Model file for the job. Use its own axes, mm. Round coordinates to 2 decimals unless told otherwise and drop trailing zeros. Loops run counter-clockwise (first coordinate to the right, second up) from the corner with the lowest first, then second, coordinate; pieces in that order, holes last. Notation, with made-up numbers: M 79.5,17 L 115.5,17 A19 cw 115.5,47 Z; hole C -10.5,-22 d2. An arc over 180 degrees is marked long. Use a Markdown table: item, result. Add a question column.
Item 1: Saw through at A-A on z = 2.5. Write the cut outline in (x, y), then the cut area to 3 significant figures.
Item 2: Pin check, flat tips, straight feed: P1, Ø1.2, axis at x = -10, y = 10.5, coming from the +Z side; P2, Ø1.5, axis at x = -10.86, y = 11.26, coming from the +Z side; P3, Ø4, axis at y = 7.5, z = 2, coming from the +X side; P4, Ø1.5, axis at x = 12, z = 6.5, coming from the -Y side. Stop position of each tip, or through.
Item 3: Saw through at B-B on x = -10.5. Write the cut outline in (y, z).
Item 4: Saw through at D-D on y = 5.5. Write the cut outline in (x, z).
Item 5: Saw through at C-C on z = 7.5. Write the cut outline in (x, y).
Item 6: Wall check: L1, parallel to X at y = 12.5, z = 7.75; L2, parallel to X at y = 11, z = 1.75; L3, parallel to Y at x = 20, z = 5.75. Give the ranges that are in metal, low to high. Write a range as from..to.
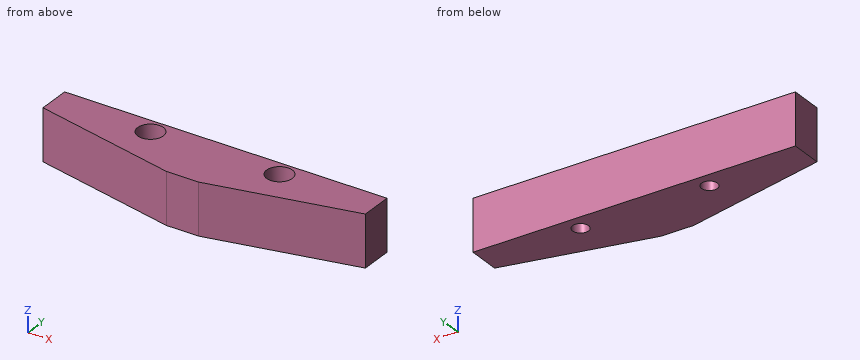
```python
from build123d import *

# Parameters (mm, degrees)
EXTRUDE_1_DEPTH     = 8
SKETCH_2_R          = 1.25
CUT_EXTRUDE_1_DEPTH = 8
SKETCH_3_R          = 2
CUT_EXTRUDE_2_DEPTH = 4


with BuildPart() as part:
    # Эскиз1 → Бобышка-Вытянуть1 (new body)
    with BuildSketch(Plane.XY):
        Polygon((-25.856072272, 13.757630696), (24.143927728, 13.757630696), (24.143927728, 8.757630696), (1.643927728, 3.757630696), (-3.356072272, 3.757630696), (-25.856072272, 8.757630696), align=None)
    extrude(amount=EXTRUDE_1_DEPTH)

    # Эскиз2 → Вырез-Вытянуть1 (cut)
    with BuildSketch(Plane.XY.offset(8)):
        with Locations((-10.856072272, 11.257630696)):
            Circle(SKETCH_2_R)
        with Locations((9.143927728, 11.257630696)):
            Circle(SKETCH_2_R)
    extrude(amount=-CUT_EXTRUDE_1_DEPTH, mode=Mode.SUBTRACT)

    # Эскиз3 → Вырез-Вытянуть2 (cut)
    with BuildSketch(Plane.XY.offset(8)):
        with Locations((-10.856072272, 11.257630696)):
            Circle(SKETCH_3_R)
        with Locations((9.143927728, 11.257630696)):
            Circle(SKETCH_3_R)
    extrude(amount=-CUT_EXTRUDE_2_DEPTH, mode=Mode.SUBTRACT)


solid = part.part
```
Entries:
| question | item | result |
|---|---|---|
| 1 | outline | M -25.86,8.76 L -3.36,3.76 L 1.64,3.76 L 24.14,8.76 L 24.14,13.76 L -25.86,13.76 Z; hole C -10.86,11.26 d2.5; hole C 9.14,11.26 d2.5 |
| 1 | area | 378 mm2 |
| 2 | P1 | z = 4 |
| 2 | P2 | through |
| 2 | P3 | x = 24.14 |
| 2 | P4 | y = 5.89 |
| 3 | outline | M 5.35,0 L 10.06,0 L 10.06,4 L 9.29,4 L 9.29,8 L 5.35,8 Z; M 12.46,0 L 13.76,0 L 13.76,8 L 13.23,8 L 13.23,4 L 12.46,4 Z |
| 4 | outline | M -11.2,0 L 9.48,0 L 9.48,8 L -11.2,8 Z |
| 5 | outline | M -25.86,8.76 L -3.36,3.76 L 1.64,3.76 L 24.14,8.76 L 24.14,13.76 L -25.86,13.76 Z; hole C -10.86,11.26 d4; hole C 9.14,11.26 d4 |
| 6 | L1 | -25.86..-12.42, -9.29..7.58, 10.71..24.14 |
| 6 | L2 | -25.86..-12.08, -9.63..7.92, 10.37..24.14 |
| 6 | L3 | 7.84..13.76 |
